Geometry check sheet. Reference: the model listing, model coordinates, mm. Round coordinates to 2 decimals unless told otherwise and drop trailing zeros. Order: outer loops, then holes, each group sorted by start corner. A loop starts at its lowest first (then second) coordinate and runs counter-clockwise, first axis right, second up. Notation, with made-up numbers: (-38, -5) - (16, -5) arc R25 ccw to (16, 25) - close; hole circle Ø6 at (-37.5, -30.5). An arc over 180 degrees is marked (long way). Return JSON: item names as keys, results as strings. Group by question number.
Q1. Sectioned sample at C-C, the plane z = 0. Record the cut outline in (x, y).
Q2. Gauge pin test, flat end, axial feed: pin 1 Ø2 at (x, z) = (30, 4) entering from -Y. Record the tip position at first contact, or that the pin passes through.
Q3. Sectioned sample at D-D, the plane x = 5. Record the cut outline in (y, z), then the cut area to 4 significant figures.
Q4. Sectioned sample at A-A, the plane y = 2.2. Record the cut outline in (x, z), then the cut area to 3 significant figures.
Q5. Material ranges on line 1 along X through (y, z) = (3.15, -4); line 2 along X through (y, z) = (1.15, 0); line 3 along X through (y, z) = (3.35, -6.25), recorded low to high.
Q6. Sectioned sample at B-B, the plane x = -30. Record the cut outline in (y, z), then the cut area to 3 significant figures.
Q7. Draft check along X on faces 1 (the flat face through (0, 0, 0)), 2 (the cylindrical face through (-34.4, 2.22, 6.93)), 3 (the cylindrical face through (-28.946, 2.218, 4.672)). Enter one of: pulls with the +X half, pulls with the -X half, needs draft (parallel to the pull), parting line crosses it, or undercut.
```python
from build123d import *

# Parameters (mm, degrees)
SKETCH_1_R      = 1.25
EXTRUDE_1_DEPTH = 4.5


with BuildPart() as part:
    # 草图1 → 凸台-拉伸1 (new body)
    with BuildSketch(Plane(origin=(0, 0, 0), x_dir=(1, 0, 0), z_dir=(0, 1, 0))):
        with BuildLine():
            Line((-33, 7.5), (33, 7.5))
            ThreePointArc((33, 7.5), (34.414213562, 6.914213562), (35, 5.5))
            Line((35, 5.5), (35, -5.5))
            ThreePointArc((35, -5.5), (34.414213562, -6.914213562), (33, -7.5))
            Line((33, -7.5), (-33, -7.5))
            ThreePointArc((-33, -7.5), (-34.414213562, -6.914213562), (-35, -5.5))
            Line((-35, -5.5), (-35, 5.5))
            ThreePointArc((-35, 5.5), (-34.414213562, 6.914213562), (-33, 7.5))
        make_face()
        with Locations(Location((-5, 0, 0), (0, 0, 270))):
            Circle(SKETCH_1_R, mode=Mode.SUBTRACT)
        with Locations(Location((5, 0, 0), (0, 0, 270))):
            Circle(SKETCH_1_R, mode=Mode.SUBTRACT)
        with Locations(Location((-30, 4, 0), (0, 0, 270))):
            Circle(SKETCH_1_R, mode=Mode.SUBTRACT)
        with Locations(Location((-30, -4, 0), (0, 0, 270))):
            Circle(SKETCH_1_R, mode=Mode.SUBTRACT)
        with Locations(Location((30, -4, 0), (0, 0, 270))):
            Circle(SKETCH_1_R, mode=Mode.SUBTRACT)
        with Locations(Location((30, 4, 0), (0, 0, 270))):
            Circle(SKETCH_1_R, mode=Mode.SUBTRACT)
    extrude(amount=EXTRUDE_1_DEPTH)


solid = part.part
```
Reply:
{
 "1": {"outline": "(-35, 0) - (-6.25, 0) - (-6.25, 4.5) - (-35, 4.5) - close; (-3.75, 0) - (3.75, 0) - (3.75, 4.5) - (-3.75, 4.5) - close; (6.25, 0) - (35, 0) - (35, 4.5) - (6.25, 4.5) - close"},
 "2": {"pin 1": "through"},
 "3": {"outline": "(0, -7.5) - (4.5, -7.5) - (4.5, -1.25) - (0, -1.25) - close; (0, 1.25) - (4.5, 1.25) - (4.5, 7.5) - (0, 7.5) - close", "area": "56.25 mm^2"},
 "4": {"outline": "(-35, -5.5) arc R2 ccw to (-33, -7.5) - (33, -7.5) arc R2 ccw to (35, -5.5) - (35, 5.5) arc R2 ccw to (33, 7.5) - (-33, 7.5) arc R2 ccw to (-35, 5.5) - close; hole circle Ø2.5 at (-30, -4); hole circle Ø2.5 at (-30, 4); hole circle Ø2.5 at (-5, 0); hole circle Ø2.5 at (5, 0); hole circle Ø2.5 at (30, -4); hole circle Ø2.5 at (30, 4)", "area": "1,020 mm^2"},
 "5": {"line 1": "-35 to -31.25, -28.75 to 28.75, 31.25 to 35", "line 2": "-35 to -6.25, -3.75 to 3.75, 6.25 to 35", "line 3": "-34.85 to 34.85"},
 "6": {"outline": "(0, -7.5) - (4.5, -7.5) - (4.5, -5.25) - (0, -5.25) - close; (0, -2.75) - (4.5, -2.75) - (4.5, 2.75) - (0, 2.75) - close; (0, 5.25) - (4.5, 5.25) - (4.5, 7.5) - (0, 7.5) - close", "area": "45.0 mm^2"},
 "7": {"face 1": "needs draft", "face 2": "pulls with the -X half", "face 3": "undercut"}
}
